Input: part model. Units: mm. Frame: model coordinates. Give positions to 0.01 mm unless a question says otherwise; leave off trailing zeros. Write each loop counter-clockwise with the first axis right and the second up, starting at its lowest first coordinate (ties: lowest second). Pieces come first, ordered by that corner, then holes. Notation, with made-up numbers: (-34, -29.75) -> (-24, -29.75) arc R34 cw to (-24, 8.25) -> close; hole circle Ø1 at (-34.5, 64.25). An arc over 180 degrees is marked (long way). Return JSON: item names as keys, results as strings. Group by question number.
Item 1: Section A-A, the plane x = 27. Return loops of the section in (y, z) (1 decimal), then the cut area to 3 significant figures.
Item 2: Pin query (flat end, axial travel): P1, Ø20.5, axis at y = 20, z = 1168, coming from the -X side; P2, Ø9.5, axis at x = 20.5, z = 1168, coming from the +Y side; P3, Ø12.5, axis at x = 21.5, z = 1177, coming from the -Y side. Return the tip coordinate at first contact, or that it passes through.
Item 3: Line query: line 1 (X direction, y = 29, z = -667); line 2 (Z direction, x = 4.5, y = 23). Output: solid intervals per line, ascending. Write a range as [from, to].
Item 4: Section C-C, the plane z = -17. Return loops of the section in (x, y), then the cut area to 3 significant figures.
from build123d import *

# Parameters (mm, degrees)
SKETCH1_W           = 50.799956
SKETCH1_H           = 50.799956
SKETCH1_W_2         = 41.274956
SKETCH1_H_2         = 41.274956
BASETUBE_DEPTH      = 1143
BOSS_EXTRUDE2_START = 1143
SKETCH1_3_W         = 41.274956
SKETCH1_3_H         = 41.274956
SKETCH1_3_W_2       = 31.749956
SKETCH1_3_H_2       = 31.749956
BOSS_EXTRUDE2_DEPTH = 50.8


with BuildPart() as part:
    # Sketch1 → BaseTube (new, symmetric)
    with BuildSketch(Plane.XY):
        with Locations((25.399978, 25.399978)):
            Rectangle(SKETCH1_W, SKETCH1_H)
        with Locations((25.399978, 25.399978)):
            Rectangle(SKETCH1_W_2, SKETCH1_H_2, mode=Mode.SUBTRACT)
    extrude(amount=BASETUBE_DEPTH, both=True)

    # Sketch1<3> → Boss-Extrude2 (add, symmetric)
    with BuildSketch(Plane.XY.offset(BOSS_EXTRUDE2_START)):
        with Locations((25.399978, 25.399978)):
            Rectangle(SKETCH1_3_W, SKETCH1_3_H)
        with Locations((25.399978, 25.399978)):
            Rectangle(SKETCH1_3_W_2, SKETCH1_3_H_2, mode=Mode.SUBTRACT)
    extrude(amount=BOSS_EXTRUDE2_DEPTH, both=True)


solid = part.part
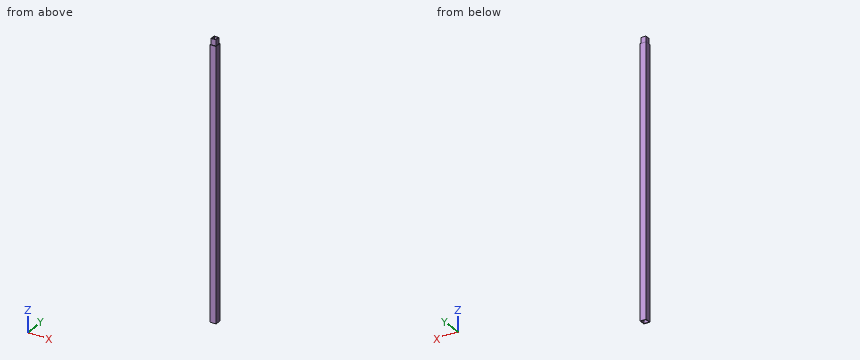
Answer below:
{
 "1": {"outline": "(0, -1143) -> (4.8, -1143) -> (4.8, 1092.2) -> (9.5, 1092.2) -> (9.5, 1193.8) -> (4.8, 1193.8) -> (4.8, 1143) -> (0, 1143) -> close; (41.3, 1092.2) -> (46, 1092.2) -> (46, -1143) -> (50.8, -1143) -> (50.8, 1143) -> (46, 1143) -> (46, 1193.8) -> (41.3, 1193.8) -> close", "area": "22,700 mm2"},
 "2": {"P1": "stops at x = 4.76", "P2": "stops at y = 46.04", "P3": "stops at y = 4.76"},
 "3": {"line 1": "x = [0, 4.76], [46.04, 50.8]", "line 2": "z = [-1143, 1143]"},
 "4": {"outline": "(0, 0) -> (50.8, 0) -> (50.8, 50.8) -> (0, 50.8) -> close; hole (4.76, 4.76) -> (46.04, 4.76) -> (46.04, 46.04) -> (4.76, 46.04) -> close", "area": "877 mm2"}
}
